The model under review builds one solid part; all positions refer to its coordinate system, in mm. Face numbers are marked on the shaded views. A direction names the side the tool comes from. Coordinates: 2 decimals unless noted, no trailing zeros. Write each loop counter-clockwise with the first axis right and the second up, starting at its lowest first coordinate (ties: lowest second). Pieces come first, ordered by that corner, then holes. Notation, with made-up numbers: (62, 16.25) - (102, 16.25) arc R30 ccw to (102, 51.25) - close; hole circle Ø11 at (-6, -20.5). An arc over 180 degrees is marked (long way). Return JSON: item names as keys, results as strings. Group by question number.
(1) We need section B-B on z = 16. State the section outline as (x, y) points, then the cut area to 3 significant figures.
(2) We need section A-A on x = -14.5. State the section outline as (y, z) points.
(3) Draft analysis for pull direction X (two halves, no side actions). For the marked faces 1, 2 and 3, state which applies: released by +X, released by -X, zero draft, split by the parting line, or undercut.
(4) Tool access review of the marked faces 4 and 5: name each direction out of +Z, -Z, +X, -X, +Y, -Y from which nothing blocks a thin tool from reaching the whole face with its end or side.
(5) We need section D-D on y = 20. Give the number of separate pieces and of enclosed holes in the cut face, then the cut area to 3 significant figures.
(6) We need section C-C on z = 30. State the section outline as (x, y) points.
(7) To check wall thickness, follow L1, parallel to Z at x = -80, y = 36.3; L2, parallel to X at y = 35, z = -4; L3, parallel to Z at x = -51, y = 6. State the ranges of each line that lie inside material, in increasing order. Write a range as from..to.
(8) For pin 1 Ø3 at (x, y) = (-82, 27) entering from +Z, flat-tipped, find the tip position at first contact; note if it passes through.
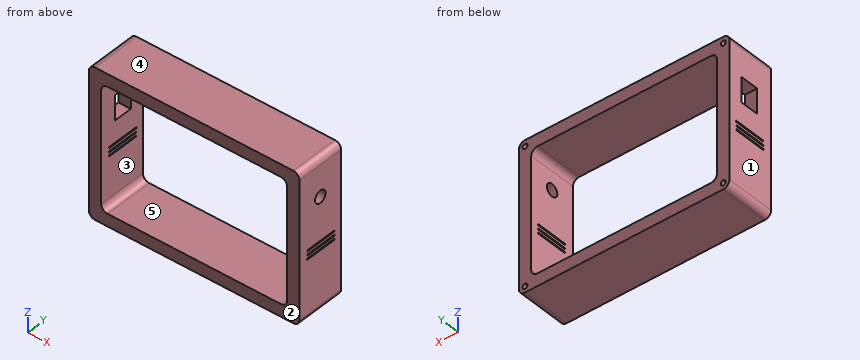
```python
from build123d import *

# Parameters (mm, degrees)
SKETCH1_W                 = 170
SKETCH1_H                 = 120
SKETCH1_W_2               = 150
SKETCH1_H_2               = 100
EXTRUDE_THIN1_DEPTH       = 40
SKETCH2_R                 = 5
CUT_EXTRUDE1_DEPTH        = 10
F_4_0MM_DOWEL_HOLE1_D     = 4
F_4_0MM_DOWEL_HOLE1_DEPTH = 5
F_4_0MM_DOWEL_HOLE1_TIP   = 1.201721238
F_4_0MM_DOWEL_HOLE2_D     = 4
F_4_0MM_DOWEL_HOLE2_DEPTH = 5
F_4_0MM_DOWEL_HOLE2_TIP   = 1.201721238
F_4_0MM_DOWEL_HOLE3_D     = 4
F_4_0MM_DOWEL_HOLE3_DEPTH = 5
F_4_0MM_DOWEL_HOLE3_TIP   = 1.201721238
F_4_0MM_DOWEL_HOLE4_D     = 4
F_4_0MM_DOWEL_HOLE4_DEPTH = 5
F_4_0MM_DOWEL_HOLE4_TIP   = 1.201721238
SKETCH15_W                = 20
SKETCH15_H                = 15
CUT_EXTRUDE7_DEPTH        = 10
FILLET1_R                 = 5
SKETCH16_W                = 1
SKETCH16_H                = 26
CUT_EXTRUDE8_DEPTH        = 1
CUT_EXTRUDE8_DEPTH_BACK   = 171
SKETCH17_W                = 1
SKETCH17_H                = 26
CUT_EXTRUDE9_DEPTH        = 1
CUT_EXTRUDE9_DEPTH_BACK   = 171
SKETCH19_W                = 1
SKETCH19_H                = 26
CUT_EXTRUDE10_DEPTH       = 1
CUT_EXTRUDE10_DEPTH_BACK  = 171
FILLET2_R                 = 5


with BuildPart() as part:
    # Sketch1 → Extrude-Thin1 (new body)
    with BuildSketch(Plane(origin=(0, 0, 0), x_dir=(1, 0, 0), z_dir=(0, 1, 0))):
        Rectangle(SKETCH1_W, SKETCH1_H)
        Rectangle(SKETCH1_W_2, SKETCH1_H_2, mode=Mode.SUBTRACT)
    extrude(amount=EXTRUDE_THIN1_DEPTH)

    # Sketch2 → Cut-Extrude1 (cut)
    with BuildSketch(Plane(origin=(85, 0, 0), x_dir=(0, 0, -1), z_dir=(1, 0, 0))):
        with Locations((-30, 20)):
            Circle(SKETCH2_R)
    extrude(amount=-CUT_EXTRUDE1_DEPTH, mode=Mode.SUBTRACT)

    # Ø4.0mm Dowel Hole1
    with Locations(Plane(origin=(0, 40, 0), x_dir=(1, 0, 0), z_dir=(0, 1, 0))):
        with Locations((-80, 55)):
            Hole(F_4_0MM_DOWEL_HOLE1_D / 2, depth=F_4_0MM_DOWEL_HOLE1_DEPTH)
            with Locations((0, 0, -(F_4_0MM_DOWEL_HOLE1_DEPTH + F_4_0MM_DOWEL_HOLE1_TIP / 2))):  # 118° drill point
                Cone(0, F_4_0MM_DOWEL_HOLE1_D / 2, F_4_0MM_DOWEL_HOLE1_TIP, mode=Mode.SUBTRACT)

    # Ø4.0mm Dowel Hole2
    with Locations(Plane(origin=(0, 40, 0), x_dir=(1, 0, 0), z_dir=(0, 1, 0))):
        with Locations((-80, -55)):
            Hole(F_4_0MM_DOWEL_HOLE2_D / 2, depth=F_4_0MM_DOWEL_HOLE2_DEPTH)
            with Locations((0, 0, -(F_4_0MM_DOWEL_HOLE2_DEPTH + F_4_0MM_DOWEL_HOLE2_TIP / 2))):  # 118° drill point
                Cone(0, F_4_0MM_DOWEL_HOLE2_D / 2, F_4_0MM_DOWEL_HOLE2_TIP, mode=Mode.SUBTRACT)

    # Ø4.0mm Dowel Hole3
    with Locations(Plane(origin=(0, 40, 0), x_dir=(1, 0, 0), z_dir=(0, 1, 0))):
        with Locations((80, -55)):
            Hole(F_4_0MM_DOWEL_HOLE3_D / 2, depth=F_4_0MM_DOWEL_HOLE3_DEPTH)
            with Locations((0, 0, -(F_4_0MM_DOWEL_HOLE3_DEPTH + F_4_0MM_DOWEL_HOLE3_TIP / 2))):  # 118° drill point
                Cone(0, F_4_0MM_DOWEL_HOLE3_D / 2, F_4_0MM_DOWEL_HOLE3_TIP, mode=Mode.SUBTRACT)

    # Ø4.0mm Dowel Hole4
    with Locations(Plane(origin=(0, 40, 0), x_dir=(1, 0, 0), z_dir=(0, 1, 0))):
        with Locations((80, 55)):
            Hole(F_4_0MM_DOWEL_HOLE4_D / 2, depth=F_4_0MM_DOWEL_HOLE4_DEPTH)
            with Locations((0, 0, -(F_4_0MM_DOWEL_HOLE4_DEPTH + F_4_0MM_DOWEL_HOLE4_TIP / 2))):  # 118° drill point
                Cone(0, F_4_0MM_DOWEL_HOLE4_D / 2, F_4_0MM_DOWEL_HOLE4_TIP, mode=Mode.SUBTRACT)

    # Sketch15 → Cut-Extrude7 (cut)
    with BuildSketch(Plane.ZY.offset(85)):
        with Locations((22.837644719, 20.840649499)):
            Rectangle(SKETCH15_W, SKETCH15_H)
    extrude(amount=-CUT_EXTRUDE7_DEPTH, mode=Mode.SUBTRACT)

    # Fillet1
    fillet1_edges = [part.edges().sort_by_distance(p)[0] for p in [
        (85, 20, 60),
        (-85, 20, 60),
        (-85, 20, -60),
        (85, 20, -60),
    ]]
    fillet(fillet1_edges, radius=FILLET1_R)

    # Sketch16 → Cut-Extrude8 (cut, two sides)
    with BuildSketch(Plane(origin=(85, 0, 0), x_dir=(0, 0, -1), z_dir=(1, 0, 0))) as cut_extrude8_sk:
        with Locations((5.123572244, 20.634211022)):
            Rectangle(SKETCH16_W, SKETCH16_H)
    extrude(amount=CUT_EXTRUDE8_DEPTH, mode=Mode.SUBTRACT)
    extrude(cut_extrude8_sk.sketch, amount=-CUT_EXTRUDE8_DEPTH_BACK, mode=Mode.SUBTRACT)

    # Sketch17 → Cut-Extrude9 (cut, two sides)
    with BuildSketch(Plane(origin=(85, 0, 0), x_dir=(0, 0, -1), z_dir=(1, 0, 0))) as cut_extrude9_sk:
        with Locations((8.466927988, 20.476753878)):
            Rectangle(SKETCH17_W, SKETCH17_H)
    extrude(amount=CUT_EXTRUDE9_DEPTH, mode=Mode.SUBTRACT)
    extrude(cut_extrude9_sk.sketch, amount=-CUT_EXTRUDE9_DEPTH_BACK, mode=Mode.SUBTRACT)

    # Sketch19 → Cut-Extrude10 (cut, two sides)
    with BuildSketch(Plane(origin=(85, 0, 0), x_dir=(0, 0, -1), z_dir=(1, 0, 0))) as cut_extrude10_sk:
        with Locations((11.568551735, 20.390257517)):
            Rectangle(SKETCH19_W, SKETCH19_H)
    extrude(amount=CUT_EXTRUDE10_DEPTH, mode=Mode.SUBTRACT)
    extrude(cut_extrude10_sk.sketch, amount=-CUT_EXTRUDE10_DEPTH_BACK, mode=Mode.SUBTRACT)

    # Fillet2
    fillet2_edges = [part.edges().sort_by_distance(p)[0] for p in [
        (75, 20, 50),
        (75, 20, -50),
        (-75, 20, -50),
        (-75, 20, 50),
    ]]
    fillet(fillet2_edges, radius=FILLET2_R)


solid = part.part
```
Ans:
{
 "1": {"outline": "(-85, 0) - (-75, 0) - (-75, 13.34) - (-85, 13.34) - close; (-85, 28.34) - (-75, 28.34) - (-75, 40) - (-85, 40) - close; (75, 0) - (85, 0) - (85, 40) - (75, 40) - close", "area": "650 mm²"},
 "2": {"outline": "(0, -60) - (40, -60) - (40, -50) - (0, -50) - close; (0, 50) - (40, 50) - (40, 60) - (0, 60) - close"},
 "3": {"face 1": "released by -X", "face 2": "zero draft", "face 3": "undercut"},
 "4": {"face 4": "+Z, +X, -X, +Y, -Y", "face 5": "+Y, -Y"},
 "5": {"separate pieces": "8", "enclosed holes": "0", "area": "5,040 mm²"},
 "6": {"outline": "(-85, 0) - (-75, 0) - (-75, 13.34) - (-85, 13.34) - close; (-85, 28.34) - (-75, 28.34) - (-75, 40) - (-85, 40) - close; (75, 0) - (85, 0) - (85, 15) - (75, 15) - close; (75, 25) - (85, 25) - (85, 40) - (75, 40) - close"},
 "7": {"L1": "-60..-57, -53..53, 57..60", "L2": "-85..-75, 75..85", "L3": "-60..-50, 50..60"},
 "8": {"pin 1": "z = 59.97"}
}
